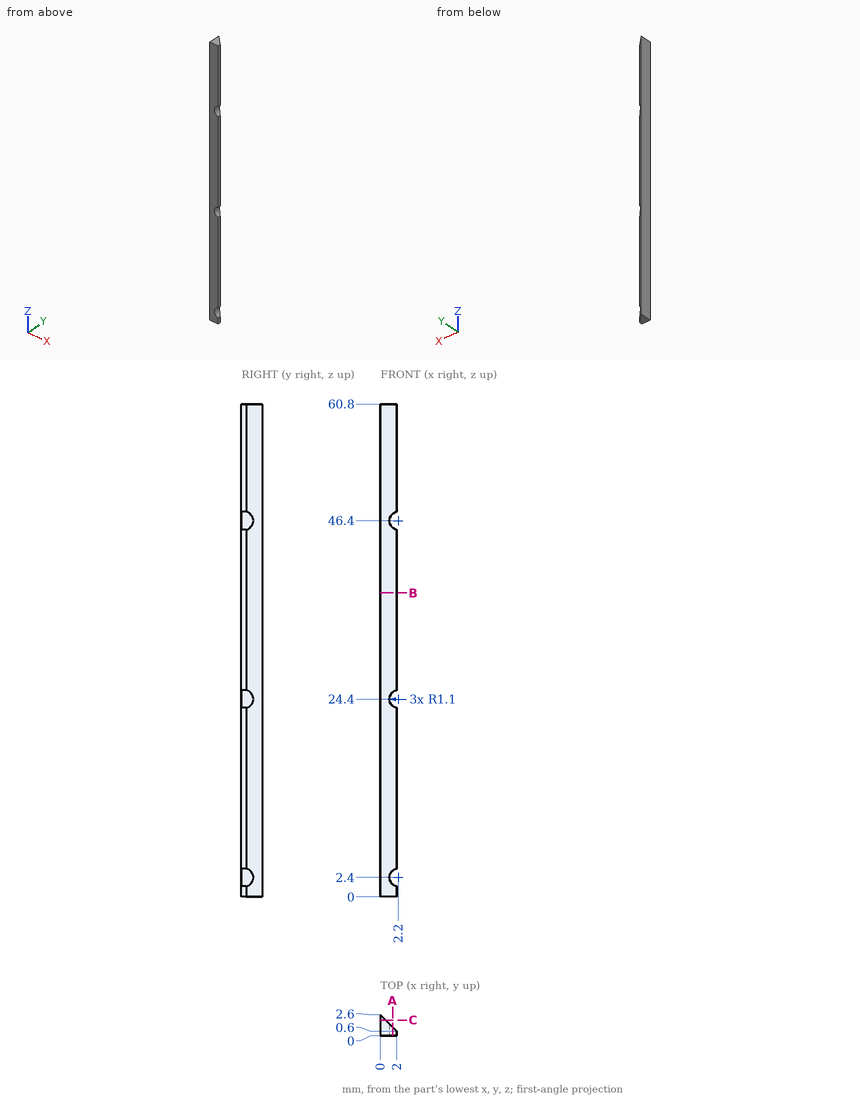
Geometry: see drawing. Coordinates: mm, zero at the bounding-box minimum. Coordinates: 2 decimals unless noted, no trailing zeros. Loops run counter-clockwise (first coordinate to the right, second up) from the corner with the lowest first, then second, coordinate; pieces in that order, holes last.
(1) Material intervals for probe 1 along Z at (x, y) = (1.85, 0.1); probe 2 along Z at (x, y) = (1.25, 0.9); probe 3 along X at (y, z) = (1.1, 37.5), sorted ascending.
(2) Section C-C on y = 1.95. Return the cut outline in (x, z).
(3) Section B-B on z = 37.5. Return the cut outline in (x, y), then the cut area to 3 significant figures.
(4) Section A-A on x = 1.5. Return the cut outline in (y, z), then the cut area to 3 significant figures.
Data:
1. probe 1: z = 0 to 1.36, 3.44 to 23.36, 25.44 to 45.36, 47.44 to 60.8
1. probe 2: z = 0 to 1.85, 2.95 to 23.85, 24.95 to 45.85, 46.95 to 60.8
1. probe 3: x = 0 to 1.5
2. outline: (0, 0) - (0.65, 0) - (0.65, 60.8) - (0, 60.8) - close
3. outline: (0, 0) - (2, 0) - (2, 0.6) - (0, 2.6) - close
3. area: 3.20 mm2
4. outline: (0, 0) - (1.1, 0) - (1.1, 1.55) - (0, 1.55) - close; (0, 3.25) - (1.1, 3.25) - (1.1, 23.55) - (0, 23.55) - close; (0, 25.25) - (1.1, 25.25) - (1.1, 45.55) - (0, 45.55) - close; (0, 47.25) - (1.1, 47.25) - (1.1, 60.8) - (0, 60.8) - close
4. area: 61.3 mm2
